Can you work these out from the model? Positions are in its coordinate system, mm. Coordinates: 2 decimals unless noted, no trailing zeros. Loops run counter-clockwise (first coordinate to the right, second up) from the corner with the lowest first, then second, coordinate; pieces in that order, holes last.
Autodesk Inventor part; units mm, degrees
ref_plane "YZ Plane" through (0, 0, 0) normal (1, 0, 0) x (0, 1, 0)
ref_plane "XZ Plane" through (0, 0, 0) normal (0, 1, 0) x (-1, 0, 0)
ref_plane "XY Plane" through (0, 0, 0) normal (0, 0, 1) x (1, 0, 0)
sketch "Sketch1" plane through (0, 0, 0) normal (0, 0, 1) x (1, 0, 0)
  line L0 (213.0422, 0) -> (106.5211, -184.5)
  line L1 (106.5211, -184.5) -> (-106.5211, -184.5)
  line L2 (-106.5211, -184.5) -> (-213.0422, 0)
  line L3 (-213.0422, 0) -> (-106.5211, 184.5)
  line L4 (-106.5211, 184.5) -> (106.5211, 184.5)
  line L5 (106.5211, 184.5) -> (213.0422, 0)
  point P0 (0, 0)
  point P1 (0, 0)
  dimension "d0" = 369
extrude "Extrusion1" add sketch "Sketch1" along normal blind 3
sketch "Sketch3" plane through (0, 0, 3) normal (0, 0, 1) x (1, 0, 0)
  line L0 (20.9, -20.75) -> (20.9, 20.75)
  arc A0 (17.5, -24.15) -> (20.9, -20.75) centre (17.5, -20.75) ccw
  line L1 (-17.5, -24.15) -> (17.5, -24.15)
  arc A1 (-20.9, -20.75) -> (-17.5, -24.15) centre (-17.5, -20.75) ccw
  line L2 (-20.9, 20.75) -> (-20.9, -20.75)
  arc A2 (-17.5, 24.15) -> (-20.9, 20.75) centre (-17.5, 20.75) ccw
  line L3 (17.5, 24.15) -> (-17.5, 24.15)
  arc A3 (20.9, 20.75) -> (17.5, 24.15) centre (17.5, 20.75) ccw
  line L4 (213.6196, 0) -> (106.8098, -185)
  line L5 (106.8098, 185) -> (213.6196, 0)
  line L6 (-106.8098, 185) -> (106.8098, 185)
  line L7 (-213.6196, 0) -> (-106.8098, 185)
  line L8 (-106.8098, -185) -> (-213.6196, 0)
  line L9 (106.8098, -185) -> (-106.8098, -185)
  point P0 (0, 0)
extrude "Extrusion2" cut sketch "Sketch3" against normal blind 3 contours A0 L1 A1 L2 A2 L3 A3 L0
sketch "Sketch4" plane through (0, 0, 0) normal (0, 0, -1) x (-1, 0, 0)
  line L0 (49.5995, 87.1474) -> (49.5995, -46.8)
  line L1 (48.3995, -48) -> (-73.3995, -48)
  line L2 (-74.5995, -46.8) -> (-74.5995, 87.1474)
  arc A0 (-39.8967, 142.8769) -> (-74.5995, 87.1474) centre (-12.5, 87.1474) ccw
  arc A1 (49.5995, 87.1474) -> (14.8967, 142.8769) centre (-12.5, 87.1474) ccw
  line L3 (-82.5, -56) -> (57.5, -56)
  line L4 (57.5, -56) -> (57.5, 151)
  line L5 (57.5, 151) -> (-82.5, 151)
  line L6 (-82.5, 151) -> (-82.5, -56)
  line L7 (-39.8967, 142.8769) -> (14.8967, 142.8769)
  point P0 (0, 0)
  dimension "d5" = 140
  dimension "d6" = 207
  dimension "d8" = 57.5
  dimension "d11" = 56
extrude "Extrusion3" cut sketch "Sketch4" against normal blind 1
properties part number "AEON.AcrylicTop"
(1) If I drill on probe 1 along Y at (x, z) = (14, 1.35); probe 2 along Y at (x, z) = (31.5, 0.95); probe 3 along Z at (x, y) = (75, 42.5), over which ranges is the centre line in solid material (lowest first)?
Check values:
probe 1: y = -184.5 to -24.15, 24.15 to 184.5
probe 2: y = -184.5 to -56, 151 to 184.5
probe 3: z = 1 to 3
(2) I want a section at C-C on x = 62. Write out the boundary of the cut face in (y, z), then the cut area to 3 significant figures.
Check values:
outline: (-184.5, 0) - (-56, 0) - (-56, 1) - (151, 1) - (151, 0) - (184.5, 0) - (184.5, 3) - (-184.5, 3) - close
area: 900 mm2
(3) I'm going to push flat-ended pins straight in: pin 1 (1 mm diameter, centred on y = -4.5, z = 2, fed in from -X); pin 2 (1.5 mm diameter, centred on x = 107.5, z = 2.5, fed in from +Y); pin 3 (1.6 mm diameter, centred on y = -9.5, z = 2.5, fed in from +X). Where does each tip first touch, or does it pass through?
Check values:
pin 1: stops at x = -210.73
pin 2: stops at y = 184.1
pin 3: stops at x = 208.02
(4) I want a section at D-D on y = -10. Write out the boundary of the cut face in (x, z), then the cut area to 3 significant figures.
Check values:
outline: (-207.27, 0) - (-57.5, 0) - (-57.5, 1) - (-20.9, 1) - (-20.9, 3) - (-207.27, 3) - close; (20.9, 1) - (82.5, 1) - (82.5, 0) - (207.27, 0) - (207.27, 3) - (20.9, 3) - close
area: 1,020 mm2
(5) If we mould it in two halves opening along X, with no side actions, what happens to faces 1 (the flat face through (13, 49, 1)), 2 (the flat face through (-159.036, -93.541, 1.479)), 3 (the flat face through (160.527, -90.959, 1.479))? For each: released by +X, released by -X, zero draft, split by the parting line, or undercut.
Check values:
face 1: undercut
face 2: released by -X
face 3: released by +X
(6) I want a section at A-A on z = 1.95. Write out the boundary of the cut face in (x, y).
Check values:
outline: (-213.04, 0) - (-106.52, -184.5) - (106.52, -184.5) - (213.04, 0) - (106.52, 184.5) - (-106.52, 184.5) - close; hole (-20.9, -20.75) arc R3.4 ccw to (-17.5, -24.15) - (17.5, -24.15) arc R3.4 ccw to (20.9, -20.75) - (20.9, 20.75) arc R3.4 ccw to (17.5, 24.15) - (-17.5, 24.15) arc R3.4 ccw to (-20.9, 20.75) - close
(7) I want a section at B-B on y = 95. Write out the boundary of the cut face in (x, z), then the cut area to 3 significant figures.
Check values:
outline: (-158.19, 0) - (-57.5, 0) - (-57.5, 1) - (82.5, 1) - (82.5, 0) - (158.19, 0) - (158.19, 3) - (-158.19, 3) - close
area: 809 mm2
